Work out the finished part from the listing and answer in its coordinate system (mm). Face numbers are marked on the shaded views. Coordinates: 2 decimals unless noted, no trailing zeros. Write each loop counter-clockwise with the first axis right and the second up, starting at its lowest first coordinate (ties: lowest second). Pieces come first, ordered by that corner, then holes. Notation, with made-up numbers: (61.25, 46.5) - (99.25, 46.5) arc R28 ccw to (99.25, 73.5) - close; hole circle Ø7 at (-29.75, -26.5). An arc over 180 degrees is marked (long way). One line per item, written item: value.
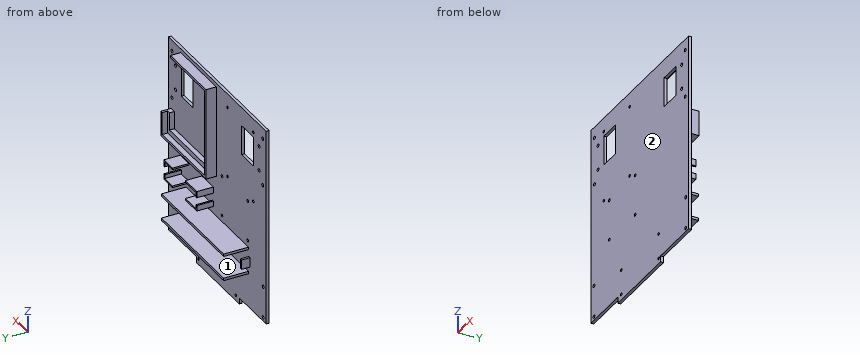
```python
from build123d import *

# Parameters (mm, degrees)
SKETCH_1_W           = 220
SKETCH_1_H           = 240
EXTRUDE_2_DEPTH      = 3.5
SKETCH_2_R           = 2
CUT_EXTRUDE_2_DEPTH  = 3.5
SKETCH_3_R           = 2
CUT_EXTRUDE_3_DEPTH  = 3.5
SKETCH_5_R           = 1.6
CUT_EXTRUDE_4_DEPTH  = 5
EXTRUDE_5_DEPTH      = 6
EXTRUDE_6_DEPTH      = 6.5
EXTRUDE_6_DEPTH_BACK = 6.6
SKETCH_10_R          = 1.6
CUT_EXTRUDE_5_DEPTH  = 6.5
SKETCH_11_W          = 140
SKETCH_11_H          = 3
EXTRUDE_7_DEPTH      = 30
SKETCH_12_W          = 3.232393119
SKETCH_12_H          = 20.299160217
EXTRUDE_8_DEPTH      = 10
SKETCH_13_W          = 2.764768701
SKETCH_13_H          = 11.651525239
EXTRUDE_9_DEPTH      = 10
SKETCH_16_W          = 96.137938664
SKETCH_16_H          = 7.416001845
EXTRUDE_10_DEPTH     = 3.5
SKETCH_17_R          = 1.6
EXTRUDE_11_DEPTH     = 3.5
SKETCH_18_R          = 1.6
CUT_EXTRUDE_7_DEPTH  = 10
SKETCH_19_R          = 1.75
CUT_EXTRUDE_8_DEPTH  = 10
SKETCH_20_W          = 74
SKETCH_20_H          = 24.3
SKETCH_20_W_2        = 70
SKETCH_20_H_2        = 20.3
EXTRUDE_12_DEPTH     = 20
SKETCH_21_W          = 74
SKETCH_21_H          = 9.741779049
CUT_EXTRUDE_9_DEPTH  = 20
SKETCH_22_W          = 29.010965049
SKETCH_22_H          = 24.3
CUT_EXTRUDE_10_DEPTH = 20
SKETCH_23_W          = 26.105014581
SKETCH_23_H          = 35.922285021
CUT_EXTRUDE_11_DEPTH = 20


with BuildPart() as part:
    # 草图1 → 凸台-拉伸2 (new body)
    with BuildSketch(Plane(origin=(0, 0, 0), x_dir=(1, 0, 0), z_dir=(0, 1, 0))):
        with Locations((0, 20)):
            Rectangle(SKETCH_1_W, SKETCH_1_H)
    extrude(amount=EXTRUDE_2_DEPTH)

    # 草图2 → 切除-拉伸2 (cut)
    with BuildSketch(Plane(origin=(0, 3.5, 0), x_dir=(1, 0, 0), z_dir=(0, 1, 0))):
        with Locations(Location((-102, -28.658278573, 0), (0, 0, 270))):
            Circle(SKETCH_2_R)
        with Locations(Location((-102, -86.658278573, 0), (0, 0, 270))):
            Circle(SKETCH_2_R)
        with Locations(Location((-94, -42.658278573, 0), (0, 0, 270))):
            Circle(SKETCH_2_R)
        with Locations(Location((-94, -72.658278573, 0), (0, 0, 270))):
            Circle(SKETCH_2_R)
        with Locations(Location((94, -72.658278573, 0), (0, 0, 90))):
            Circle(SKETCH_2_R)
        with Locations(Location((94, -42.658278573, 0), (0, 0, 90))):
            Circle(SKETCH_2_R)
        with Locations(Location((102, -86.658278573, 0), (0, 0, 90))):
            Circle(SKETCH_2_R)
        with Locations(Location((102, -28.658278573, 0), (0, 0, 90))):
            Circle(SKETCH_2_R)
    extrude(amount=-CUT_EXTRUDE_2_DEPTH, mode=Mode.SUBTRACT)

    # 草图3 → 切除-拉伸3 (cut)
    with BuildSketch(Plane(origin=(0, 3.5, 0), x_dir=(1, 0, 0), z_dir=(0, 1, 0))):
        with Locations(Location((-103.111804302, 135.498442221, 0), (0, 0, 270))):
            Circle(SKETCH_3_R)
        with Locations(Location((-103.111804302, 97.198442221, 0), (0, 0, 270))):
            Circle(SKETCH_3_R)
        with Locations(Location((103.111804302, 97.198442221, 0), (0, 0, 90))):
            Circle(SKETCH_3_R)
        with Locations(Location((103.111804302, 135.498442221, 0), (0, 0, 90))):
            Circle(SKETCH_3_R)
    extrude(amount=-CUT_EXTRUDE_3_DEPTH, mode=Mode.SUBTRACT)

    # 草图5 → 切除-拉伸4 (cut)
    with BuildSketch(Plane(origin=(0, 3.5, 0), x_dir=(1, 0, 0), z_dir=(0, 1, 0))):
        with Locations(Location((-81.020690523, 2.946124731, 0), (0, 0, 270))):
            Circle(SKETCH_5_R)
        with Locations(Location((-23.020690523, 2.946124731, 0), (0, 0, 270))):
            Circle(SKETCH_5_R)
        with Locations(Location((-81.020690523, -83.053875269, 0), (0, 0, 270))):
            Circle(SKETCH_5_R)
        with Locations(Location((-23.020690523, -83.053875269, 0), (0, 0, 270))):
            Circle(SKETCH_5_R)
    extrude(amount=-CUT_EXTRUDE_4_DEPTH, mode=Mode.SUBTRACT)

    # 草图6 → 凸台-拉伸5 (add)
    with BuildSketch(Plane(origin=(0, 3.5, 0), x_dir=(1, 0, 0), z_dir=(0, 1, 0))):
        Polygon((5.262523113, 13.061457841), (5.262523113, -92.338542159), (82.027739865, -92.338542159), (82.027739865, -87.674935575), (15.799538285, -87.674935575), (15.799538285, 7.122294137), (18.613154692, 7.122294137), (82.027739865, 7.122294137), (96.312253931, 7.122294137), (96.312253931, -14.304476962), (100.562523113, -14.304476962), (100.562523113, 13.061457841), align=None)
    extrude(amount=EXTRUDE_5_DEPTH)

    # 草图9 → 凸台-拉伸6 (add, two sides: drawn at the far end of the back side and taken through both)
    with BuildSketch(Plane(origin=(0, 9.5, 0), x_dir=(1, 0, 0), z_dir=(0, 1, 0)).offset(-EXTRUDE_6_DEPTH_BACK)):
        Polygon((100.562523113, -14.304476962), (103.562523113, -14.304476962), (103.562523113, 16.061457841), (2.262523113, 16.061457841), (2.262523113, -95.338542159), (82.027739865, -95.338542159), (82.027739865, -92.338542159), (5.262523113, -92.338542159), (5.262523113, 13.061457841), (100.562523113, 13.061457841), align=None)
    extrude(amount=EXTRUDE_6_DEPTH + EXTRUDE_6_DEPTH_BACK)

    # 草图10 → 切除-拉伸5 (cut)
    with BuildSketch(Plane(origin=(0, 3.5, 0), x_dir=(1, 0, 0), z_dir=(0, 1, 0))):
        with Locations(Location((-41.742355154, 136.315932828, 0), (0, 0, 270))):
            Circle(SKETCH_10_R)
        with Locations(Location((42.257644846, 136.315932828, 0), (0, 0, 270))):
            Circle(SKETCH_10_R)
        with Locations(Location((42.257644846, 106.015932828, 0), (0, 0, 270))):
            Circle(SKETCH_10_R)
        with Locations(Location((-41.742355154, 106.015932828, 0), (0, 0, 270))):
            Circle(SKETCH_10_R)
    extrude(amount=-CUT_EXTRUDE_5_DEPTH, mode=Mode.SUBTRACT)

    # 草图11 → 凸台-拉伸7 (add)
    with BuildSketch(Plane(origin=(0, 3.5, 0), x_dir=(1, 0, 0), z_dir=(0, 1, 0))):
        with Locations((-0.160177845, 97.161173923)):
            Rectangle(SKETCH_11_W, SKETCH_11_H)
        with Locations((-0.160177845, 67.099391039)):
            Rectangle(SKETCH_11_W, SKETCH_11_H)
    extrude(amount=EXTRUDE_7_DEPTH)

    # 草图12 → 凸台-拉伸8 (add)
    with BuildSketch(Plane(origin=(0, 3.5, 0), x_dir=(1, 0, 0), z_dir=(0, 1, 0))):
        with Locations((71.456018715, 82.21636334)):
            Rectangle(SKETCH_12_W, SKETCH_12_H)
    extrude(amount=EXTRUDE_8_DEPTH)

    # 草图13 → 凸台-拉伸9 (add)
    with BuildSketch(Plane(origin=(0, 3.5, 0), x_dir=(1, 0, 0), z_dir=(0, 1, 0))):
        with Locations((-72.199784206, 82.73648821)):
            Rectangle(SKETCH_13_W, SKETCH_13_H)
    extrude(amount=EXTRUDE_9_DEPTH)

    # 草图16 → 凸台-拉伸10 (add)
    with BuildSketch(Plane(origin=(0, 3.5, 0), x_dir=(1, 0, 0), z_dir=(0, 1, 0))):
        with Locations((-1.491522008, 143.708000922)):
            Rectangle(SKETCH_16_W, SKETCH_16_H)
    extrude(amount=-EXTRUDE_10_DEPTH)

    # 草图17 → 凸台-拉伸11 (add)
    with BuildSketch(Plane(origin=(0, 3.5, 0), x_dir=(1, 0, 0), z_dir=(0, 1, 0))):
        with Locations((-41.742355154, 136.315932828)):
            Circle(SKETCH_17_R)
        with Locations((-41.742355154, 106.015932828)):
            Circle(SKETCH_17_R)
        with Locations((42.257644846, 106.015932828)):
            Circle(SKETCH_17_R)
        with Locations((42.257644846, 136.315932828)):
            Circle(SKETCH_17_R)
    extrude(amount=-EXTRUDE_11_DEPTH)

    # 草图18 → 切除-拉伸7 (cut)
    with BuildSketch(Plane(origin=(0, 3.5, 0), x_dir=(1, 0, 0), z_dir=(0, 1, 0))):
        with Locations(Location((-41.742355154, 140.688952656, 0), (0, 0, 270))):
            Circle(SKETCH_18_R)
        with Locations(Location((-41.742355154, 110.388952656, 0), (0, 0, 270))):
            Circle(SKETCH_18_R)
        with Locations(Location((42.257644846, 110.388952656, 0), (0, 0, 270))):
            Circle(SKETCH_18_R)
        with Locations(Location((42.257644846, 140.688952656, 0), (0, 0, 270))):
            Circle(SKETCH_18_R)
    extrude(amount=-CUT_EXTRUDE_7_DEPTH, mode=Mode.SUBTRACT)

    # 草图19 → 切除-拉伸8 (cut)
    with BuildSketch(Plane(origin=(0, 3.5, 0), x_dir=(1, 0, 0), z_dir=(0, 1, 0))):
        with Locations(Location((-10.609897324, 58.100897113, 0), (0, 0, 270))):
            Circle(SKETCH_19_R)
        with Locations(Location((-68.609897324, 58.100897113, 0), (0, 0, 270))):
            Circle(SKETCH_19_R)
        with Locations(Location((-68.609897324, 9.100897113, 0), (0, 0, 270))):
            Circle(SKETCH_19_R)
        with Locations(Location((-10.609897324, 9.100897113, 0), (0, 0, 270))):
            Circle(SKETCH_19_R)
    extrude(amount=-CUT_EXTRUDE_8_DEPTH, mode=Mode.SUBTRACT)

    # 草图20 → 凸台-拉伸12 (add)
    with BuildSketch(Plane(origin=(0, 3.5, 0), x_dir=(1, 0, 0), z_dir=(0, 1, 0))):
        with Locations((45.932869354, 45.125549951)):
            Rectangle(SKETCH_20_W, SKETCH_20_H)
        with Locations((45.932869354, 45.125549951)):
            Rectangle(SKETCH_20_W_2, SKETCH_20_H_2, mode=Mode.SUBTRACT)
    extrude(amount=EXTRUDE_12_DEPTH)

    # 草图21 → 切除-拉伸9 (cut)
    with BuildSketch(Plane(origin=(0, 23.5, 0), x_dir=(1, 0, 0), z_dir=(0, 1, 0))):
        with Locations((45.932869354, 45.559941107)):
            Rectangle(SKETCH_21_W, SKETCH_21_H)
    extrude(amount=-CUT_EXTRUDE_9_DEPTH, mode=Mode.SUBTRACT)

    # 草图22 → 切除-拉伸10 (cut)
    with BuildSketch(Plane(origin=(0, 23.5, 0), x_dir=(1, 0, 0), z_dir=(0, 1, 0))):
        with Locations((49.104478838, 45.125549951)):
            Rectangle(SKETCH_22_W, SKETCH_22_H)
    extrude(amount=-CUT_EXTRUDE_10_DEPTH, mode=Mode.SUBTRACT)

    # 草图23 → 切除-拉伸11 (cut)
    with BuildSketch(Plane(origin=(0, 3.5, 0), x_dir=(1, 0, 0), z_dir=(0, 1, 0))):
        with Locations((-67.939973843, -59.515678039)):
            Rectangle(SKETCH_23_W, SKETCH_23_H)
        with Locations((67.939973843, -59.515678039)):
            Rectangle(SKETCH_23_W, SKETCH_23_H)
    extrude(amount=-CUT_EXTRUDE_11_DEPTH, mode=Mode.SUBTRACT)


solid = part.part
```
Item 1: Determine the mould class of the marked faces 1 and 2 for opening direction Z: +Z half, -Z half, draft (parallel to the pull), parting line (faces both ways), or undercut.
Evaluation:
face 1: undercut
face 2: draft
Item 2: Consider probe 1 along Z at (x, y) = (24, 15.5); probe 2 along Z at (x, y) = (1, 26); probe 3 along X at (y, z) = (16, -55.5). Determine where each line is inside the solid, lowest interval first.
Evaluation:
probe 1: z = -98.66 to -95.66, -68.6 to -65.6, -57.28 to -55.28, -34.98 to -32.98, -16.06 to -13.06, 92.34 to 95.34
probe 2: z = -98.66 to -95.66, -68.6 to -65.6
probe 3: x = 8.93 to 34.6, 63.61 to 82.93
Item 3: Given pin 1 (16 mm diameter, centred on x = 26, y = 17.5, fed in from +Z); pin 2 (10 mm diameter, centred on x = -39, z = -7, fed in from +Y); pin 3 (7.5 mm diameter, centred on y = 16.5, z = -55, fed in from -X), each flat-ended and moving along its own axis, determine where each tip first touches the part or whether it passes through.
Evaluation:
pin 1: stops at z = 95.34
pin 2: stops at y = 3.5
pin 3: stops at x = 8.93
Item 4: Section A-A, the plane y = 29 is taken. Determine the outline of the cut face in (x, z), then the cut area to 3 significant figures.
Evaluation:
outline: (-70.16, -98.66) - (69.84, -98.66) - (69.84, -95.66) - (-70.16, -95.66) - close; (-70.16, -68.6) - (69.84, -68.6) - (69.84, -65.6) - (-70.16, -65.6) - close
area: 840 mm2
